Input: part model. Units: mm. Frame: model coordinates. A direction names the side the tool comes from. Coordinates: 2 decimals unless noted, no trailing zeros. Loops run counter-clockwise (first coordinate to the right, second up) from the corner with the lowest first, then second, coordinate; pieces in that order, holes last. Notation, with made-up numbers: M 65,-10.75 L 97,-10.75 A30 cw 97,16.25 Z; hole C -29,-27.5 d5. An arc over 180 degrees is marked long. Use a Markdown table: item, result. Add a question column.
1. Pin query (flat end, axial travel): pin 1 (7 mm diameter, centred on x = -3, z = -20.5, fed in from -Y). Return the tip coordinate at first contact, or that it passes through.
2. Set-up query: faces 1 (the flat face through (0, 8, -24)), 2 (the cylindrical face through (23.5, 4.9, -35.6)). Return all of +Z, -Z, +X, -X, +Y, -Y with unobstructed straight access to the full face (end or side cutting, diameter ignored); none if empty.
3. Line query: L1, parallel to X at y = 9.5, z = 8.5; L2, parallel to Z at x = -21, y = 5.5; L3, parallel to X at y = 4.75, z = 56.9. Output: solid intervals per line, ascending. Write a range as [from, to].
4. Section A-A on x = -12.45. Output: boundary loops of the cut face in (y, z).
5. Section C-C on z = 8.5. Output: boundary loops of the cut face in (x, y).
6. Section B-B on z = -20.55. Output: boundary loops of the cut face in (x, y), then the cut area to 3 significant figures.
```python
from build123d import *

# Parameters (mm, degrees)
BOSS_EXTRUDE1_DEPTH = 10
M6_TAPPED_HOLE2_D   = 5
M6_TAPPED_HOLE5_D   = 5
SKETCH14_W          = 15.472798768
SKETCH14_H          = 14.039377176
CUT_EXTRUDE1_DEPTH  = 8
M6_TAPPED_HOLE7_D   = 5


with BuildPart() as part:
    # Sketch2 → Boss-Extrude1 (new body)
    with BuildSketch(Plane(origin=(0, 0, 0), x_dir=(1, 0, 0), z_dir=(0, 1, 0))):
        Polygon((61.04, -67.5), (-61.04, -67.5), (-61.04, 37.5), (-61.04, 44.5), (61.04, 44.5), (61.04, 37.5), align=None)
    extrude(amount=BOSS_EXTRUDE1_DEPTH)

    # M6 Tapped Hole2 (through all)
    with Locations(Plane(origin=(0, 10, 0), x_dir=(1, 0, 0), z_dir=(0, 1, 0))):
        with Locations((-21, -8.5), (21, -8.5), (21, 35.5), (-21, 35.5)):
            Hole(M6_TAPPED_HOLE2_D / 2)

    # M6 Tapped Hole5 (through all)
    with Locations(Plane(origin=(0, 10, 0), x_dir=(1, 0, 0), z_dir=(0, 1, 0))):
        with Locations((-12.45, -56.9), (12.45, -56.9)):
            Hole(M6_TAPPED_HOLE5_D / 2)

    # Sketch14 → Cut-Extrude1 (cut)
    with BuildSketch(Plane(origin=(0, 0, 0), x_dir=(-1, 0, 0), z_dir=(0, -1, 0))):
        with Locations((0, 20.55)):
            Rectangle(SKETCH14_W, SKETCH14_H)
    extrude(amount=-CUT_EXTRUDE1_DEPTH, mode=Mode.SUBTRACT)

    # M6 Tapped Hole7 (through all)
    with Locations(Plane(origin=(0, 0, 0), x_dir=(-1, 0, 0), z_dir=(0, -1, 0))):
        with Locations((0, 20.55)):
            Hole(M6_TAPPED_HOLE7_D / 2)


solid = part.part
```
Answers below:
| question | item | result |
|---|---|---|
| 1 | pin 1 | stops at y = 8 |
| 2 | face 1 | -Y |
| 2 | face 2 | +Y, -Y |
| 3 | L1 | x = [-61.04, -23.5], [-18.5, 18.5], [23.5, 61.04] |
| 3 | L2 | z = [-44.5, -38], [-33, 6], [11, 67.5] |
| 3 | L3 | x = [-61.04, -14.95], [-9.95, 9.95], [14.95, 61.04] |
| 4 | outline | M 0,-44.5 L 10,-44.5 L 10,54.4 L 0,54.4 Z; M 0,59.4 L 10,59.4 L 10,67.5 L 0,67.5 Z |
| 5 | outline | M -61.04,0 L -23.5,0 L -23.5,10 L -61.04,10 Z; M -18.5,0 L 18.5,0 L 18.5,10 L -18.5,10 Z; M 23.5,0 L 61.04,0 L 61.04,10 L 23.5,10 Z |
| 6 | outline | M -61.04,0 L -7.74,0 L -7.74,8 L -2.5,8 L -2.5,10 L -61.04,10 Z; M 2.5,8 L 7.74,8 L 7.74,0 L 61.04,0 L 61.04,10 L 2.5,10 Z |
| 6 | area | 1,090 mm² |
